Could you check a few things on this model? Use its own coordinates, in mm. Face numbers are marked on the shaded views. Round coordinates to 2 decimals unless told otherwise and drop trailing zeros. Order: outer loops, then holes, each group sorted by start corner. A loop starts at its lowest first (then second) coordinate and runs counter-clockwise, first axis right, second up. Notation, with made-up numbers: M -5,78 L 10,78 A23 cw 10,101 Z; hole C 85.25,-31 d4. An arc over 180 degrees is marked long. Write each question's results on one line, items separated by ' | '. Start each with the question number.
1. We'd pull the mould along X, two halves only. Please class the marked faces 1, 2, 3 and 4: released by +X, released by -X, zero draft, split by the parting line, or undercut.
2. Suppose I cut it at C-C on x = 2. Write out the boundary of the cut face in (y, z).
3. I'm going to push flat-ended pins straight in: pin 1 (3 mm diameter, centred on y = -1, z = -1, fed in from -X); pin 2 (12.5 mm diameter, centred on x = -5, y = 3.5, fed in from +Z). Where does each tip first touch, or does it pass through?
4. Suppose I cut it at B-B on y = -5. Write out the boundary of the cut face in (x, z), and give its area (3 significant figures).
5. Suppose I cut it at A-A on z = -2.25. Write out the boundary of the cut face in (x, y), and give its area (3 significant figures).
6. Please list where these lines run through material, in increasing order: L1, parallel to X at y = -4, z = -4.25; L2, parallel to X at y = 13.5, z = -1; L3, parallel to X at y = -3, z = -1.5.
7. Suppose I cut it at D-D on y = -20.5. Write out the boundary of the cut face in (x, z), and give its area (3 significant figures).
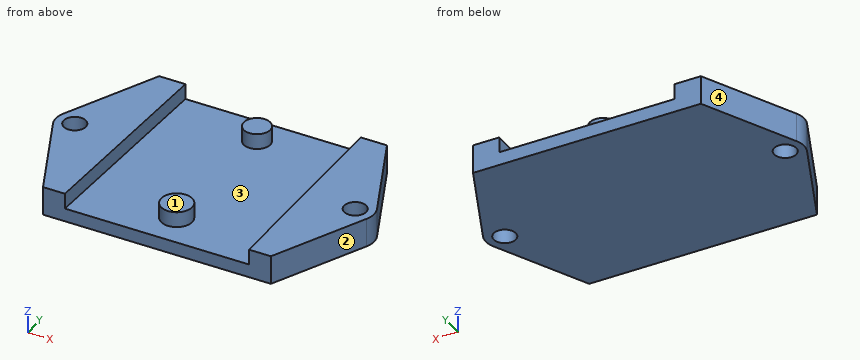
from build123d import *

# Parameters (mm, degrees)
F0_R     = 2.5
F0_R_2   = 3.5
F0_R_3   = 3
F1_DEPTH = 6.5
F2_DEPTH = 3.5
F3_R     = 5


with BuildPart() as f1:
    # F0 (on Top) → F1 (new body)
    with BuildSketch(Plane.XY):
        Polygon((-16.702011, 19.474821), (-22.702011, 19.474821), (-33.452011, -4.025179), (-22.702011, -27.525179), (-17.702011, -27.525179), align=None)
        with Locations((-28.702011, -4.025179)):
            Circle(F0_R, mode=Mode.SUBTRACT)
        Polygon((23.297989, 19.474821), (-16.702011, 19.474821), (-17.702011, -27.525179), (24.297989, -27.525179), align=None)
        with Locations((3.297989, -19.525179)):
            Circle(F0_R_2, mode=Mode.SUBTRACT)
        with Locations((3.297989, 12.974821)):
            Circle(F0_R_3, mode=Mode.SUBTRACT)
        Polygon((29.297989, 19.474821), (23.297989, 19.474821), (24.297989, -27.525179), (29.297989, -27.525179), (40.047989, -4.025179), align=None)
        with Locations((35.297989, -4.025179)):
            Circle(F0_R, mode=Mode.SUBTRACT)
        with Locations((3.297989, 12.974821)):
            Circle(F0_R_3)
        with Locations((3.297989, -19.525179)):
            Circle(F0_R_2)
    extrude(amount=-F1_DEPTH)

    # F0 (on Top) → F2 (cut)
    with BuildSketch(Plane.XY):
        Polygon((23.297989, 19.474821), (-16.702011, 19.474821), (-17.702011, -27.525179), (24.297989, -27.525179), align=None)
        with Locations((3.297989, -19.525179)):
            Circle(F0_R_2, mode=Mode.SUBTRACT)
        with Locations((3.297989, 12.974821)):
            Circle(F0_R_3, mode=Mode.SUBTRACT)
    extrude(amount=-F2_DEPTH, mode=Mode.SUBTRACT)

    # F3
    f3_edges = [f1.edges().sort_by_distance(p)[0] for p in [
        (-33.452011, -4.025179, -3.25),
        (40.047989, -4.025179, -3.25),
    ]]
    fillet(f3_edges, radius=F3_R)


solid = f1.part
Filled sheet:
1) face 1: zero draft | face 2: released by +X | face 3: undercut | face 4: released by -X
2) outline: M -27.53,-6.5 L 19.47,-6.5 L 19.47,-3.5 L 15.68,-3.5 L 15.68,0 L 10.27,0 L 10.27,-3.5 L -16.27,-3.5 L -16.27,0 L -22.78,0 L -22.78,-3.5 L -27.53,-3.5 Z
3) pin 1: stops at x = -32.72 | pin 2: stops at z = -3.5
4) outline: M -32.86,-6.5 L -31,-6.5 L -31,0 L -32.86,0 Z; M -26.4,-6.5 L 33,-6.5 L 33,0 L 23.82,0 L 23.82,-3.5 L -17.22,-3.5 L -17.22,0 L -26.4,0 Z; M 37.6,-6.5 L 39.45,-6.5 L 39.45,0 L 37.6,0 Z | area: 267 mm^2
5) outline: M -32.5,-6.11 L -22.7,-27.53 L -17.7,-27.53 L -16.7,19.47 L -22.7,19.47 L -32.5,-1.95 A5 ccw Z; C 3.3,-19.53 d7; C 3.3,12.97 d6; M 23.3,19.47 L 24.3,-27.53 L 29.3,-27.53 L 39.1,-6.11 A5 ccw 39.1,-1.95 L 29.3,19.47 Z; hole C -28.7,-4.03 d5; hole C 35.3,-4.03 d5 | area: 1,050 mm^2
6) L1: x = -32.95 to -31.2, -26.2 to 32.8, 37.8 to 39.55 | L2: x = -25.44 to -16.83, 0.34 to 6.25, 23.43 to 32.03 | L3: x = -32.85 to -30.98, -26.42 to -17.18, 23.78 to 33.02, 37.58 to 39.44
7) outline: M -25.92,-6.5 L 32.51,-6.5 L 32.51,0 L 24.15,0 L 24.15,-3.5 L 6.66,-3.5 L 6.66,0 L -0.06,0 L -0.06,-3.5 L -17.55,-3.5 L -17.55,0 L -25.92,0 Z | area: 257 mm^2
